Geometry check sheet. Reference: the model listing, model coordinates, mm. A direction names the side the tool comes from. Round coordinates to 2 decimals unless told otherwise and drop trailing zeros. Order: outer loops, then holes, each group sorted by start corner. A loop starts at its lowest first (then second) coordinate and runs counter-clockwise, first axis right, second up. Notation, with made-up numbers: (63.25, -8.75) -> (120.25, -8.75) arc R9 cw to (120.25, 5.25) -> close; hole circle Ø6 at (38.25, 69.5). An arc over 180 degrees is marked (long way). Answer as a JSON object with one key per item and string values. Group by question number.
from build123d import *

# Parameters (mm, degrees)
SKETCH1_W           = 25.4
SKETCH1_H           = 25.4
BOSS_EXTRUDE1_DEPTH = 3.175
SKETCH2_W           = 25.4
SKETCH2_H           = 3.175
BOSS_EXTRUDE2_DEPTH = 25.4
SKETCH3_R           = 4.7625
CUT_EXTRUDE1_DEPTH  = 4.175
SKETCH4_R           = 2.1971
CUT_EXTRUDE2_DEPTH  = 4.175


with BuildPart() as part:
    # Sketch1 → Boss-Extrude1 (new body)
    with BuildSketch(Plane(origin=(0, 0, 0), x_dir=(1, 0, 0), z_dir=(0, 1, 0))):
        Rectangle(SKETCH1_W, SKETCH1_H)
    extrude(amount=BOSS_EXTRUDE1_DEPTH)

    # Sketch2 → Boss-Extrude2 (add)
    with BuildSketch(Plane.XZ):
        with Locations((0, -11.1125)):
            Rectangle(SKETCH2_W, SKETCH2_H)
    extrude(amount=-BOSS_EXTRUDE2_DEPTH)

    # Sketch3 → Cut-Extrude1 (cut, through all)
    with BuildSketch(Plane(origin=(0, 3.175, 0), x_dir=(1, 0, 0), z_dir=(0, 1, 0))):
        Circle(SKETCH3_R)
    extrude(amount=-CUT_EXTRUDE1_DEPTH, mode=Mode.SUBTRACT)

    # Sketch4 → Cut-Extrude2 (cut, through all)
    with BuildSketch(Plane.XY.offset(-9.525)):
        with Locations((-6.35, 15.875)):
            Circle(SKETCH4_R)
        with Locations((6.35, 15.875)):
            Circle(SKETCH4_R)
    extrude(amount=-CUT_EXTRUDE2_DEPTH, mode=Mode.SUBTRACT)


solid = part.part
Item 1: Thickness scan on L1, parallel to Y at x = 6.35, z = -11; L2, parallel to X at y = 0.95, z = 0. Record the ranges inside material, lowest first.
Item 2: Mould release check, pull along Y, two halves, no side actions. Record for faces 3 (the flat face through (-3, 3.175, 4)), 4 (the cylindrical face through (-5.17, 17.73, -11.09)), 5 (the flat face through (12.7, 2, -5)): pulls with the +Y half, pulls with the -Y half, needs draft (parallel to the pull), parting line crosses it, or undercut.
Item 3: Sectioned sample at D-D, the plane y = 13. Enter the section's corners in (x, z) (3 decimals).
Item 4: Set-up check for faces 1 (the flat face through (0, 14, -9.525)), 2 (the flat face through (0, 25.4, -11)): record each of +Z, -Z, +X, -X, +Y, -Y from which the full face is reachable in a straight line by a thin tool's end or side.
Item 5: Depth check by flat-ended pin: pin 1 Ø11 at (x, y) = (6, 19) entering from +Z (3 decimals); pin 2 Ø10 at (x, z) = (-4.5, 5.5) entering from +Y (3 decimals). Enter the tip coordinate at first touch or a pass-through.
Item 6: Sectioned sample at A-A, the plane x = 6.35. Enter the section's corners in (y, z) (3 decimals), then the cut area to 3 significant figures.
Item 7: Sectioned sample at B-B, the plane z = 0. Enter the section's corners in (x, y) (1 decimal), then the cut area to 3 significant figures.
Item 8: Sectioned sample at C-C, the plane x = 0. Enter the section's corners in (y, z) (1 decimal), then the cut area to 3 significant figures.
Result:
{
 "1": {"L1": "y = 0 to 13.68, 18.07 to 25.4", "L2": "x = -12.7 to -4.76, 4.76 to 12.7"},
 "2": {"face 3": "pulls with the +Y half", "face 4": "undercut", "face 5": "needs draft"},
 "3": {"outline": "(-12.7, -12.7) -> (12.7, -12.7) -> (12.7, -9.525) -> (-12.7, -9.525) -> close"},
 "4": {"face 1": "+Z, +X, -X, +Y", "face 2": "+Z, -Z, +X, -X, +Y"},
 "5": {"pin 1": "stops at z = -9.525", "pin 2": "stops at y = 3.175"},
 "6": {"outline": "(0, -12.7) -> (13.678, -12.7) -> (13.678, -9.525) -> (3.175, -9.525) -> (3.175, 12.7) -> (0, 12.7) -> close; (18.072, -12.7) -> (25.4, -12.7) -> (25.4, -9.525) -> (18.072, -9.525) -> close", "area": "137 mm2"},
 "7": {"outline": "(-12.7, 0) -> (-4.8, 0) -> (-4.8, 3.2) -> (-12.7, 3.2) -> close; (4.8, 0) -> (12.7, 0) -> (12.7, 3.2) -> (4.8, 3.2) -> close", "area": "50.4 mm2"},
 "8": {"outline": "(0, -12.7) -> (25.4, -12.7) -> (25.4, -9.5) -> (3.2, -9.5) -> (3.2, -4.8) -> (0, -4.8) -> close; (0, 4.8) -> (3.2, 4.8) -> (3.2, 12.7) -> (0, 12.7) -> close", "area": "121 mm2"}
}
